Build history of the part. All positions in model axes, mm. Face numbers are marked on the shaded views. Round coordinates to 2 decimals unless told otherwise and drop trailing zeros. Loops run counter-clockwise (first coordinate to the right, second up) from the corner with the lowest first, then second, coordinate; pieces in that order, holes last. Notation, with made-up numbers: (80.5, 28) -> (126.5, 28) arc R26 ccw to (126.5, 46) -> close; hole circle Ø6 at (61, 68). An arc over 180 degrees is marked (long way). Put each result on its own line as item: value. Start each with the question number.
```python
from build123d import *


with BuildPart() as part:
    # 草图1 → 旋转1 (revolve)
    with BuildSketch(Plane.XY):
        with BuildLine():
            Line((-10, 0.5), (-5.524030949, 0.5))
            Line((-5.524030949, 0.5), (-5.170477558, 1.112372436))
            Line((-5.170477558, 1.112372436), (-4.463370777, 1.112372436))
            Line((-4.463370777, 1.112372436), (-4.30697363, 2.9))
            ThreePointArc((-4.30697363, 2.9), (-4.74222381, 3.244464966), (-4.50697363, 3.747213595))
            Line((-4.50697363, 3.747213595), (-4.50697363, 5.071428571))
            Line((-4.50697363, 5.071428571), (-3.918095147, 5.071428571))
            Line((-3.918095147, 5.071428571), (-3, 4.428571429))
            Line((-3, 4.428571429), (-3.340059177, 2.5))
            Line((-3.340059177, 2.5), (-3.840059177, 2.5))
            Line((-3.840059177, 2.5), (-4.058780836, 0))
            Line((-4.058780836, 0), (-10.5, 0))
            Line((-10.5, 0), (-11, 0.5))
            Line((-11, 0.5), (-11, 6.5))
            Line((-11, 6.5), (-10.5, 7))
            Line((-10.5, 7), (-5.170477558, 7))
            Line((-5.170477558, 7), (-5.170477558, 6.5))
            Line((-5.170477558, 6.5), (-10, 6.5))
            Line((-10, 6.5), (-10, 0.5))
        make_face()
    revolve(axis=Axis((0, 5.836193369, 0), (0, -1, 0)))


solid = part.part
```
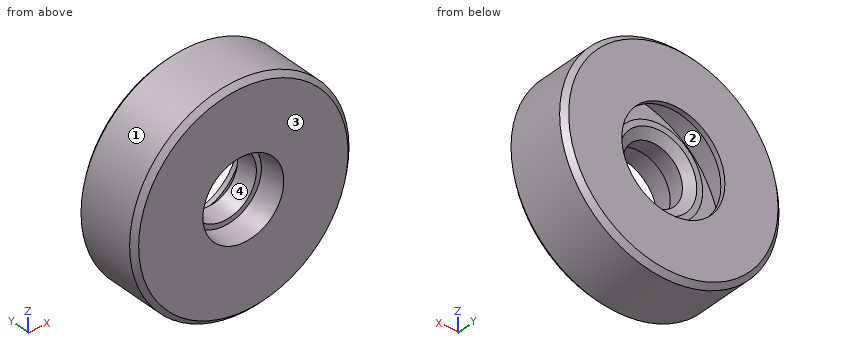
Item 1: Wall check: line 1 (X direction, y = 5.3, z = 0); line 2 (Z direction, x = -4, y = 2.25); line 3 (Y direction, x = 0.25, z = -5.75). Give the ranges that are in metal, low to high. Write a range as from..to.
Item 2: Pull direction Z, two halves, no side cores. Call the marked faces 1, 2, 3 and 4: +Z half, -Z half, draft (parallel to the pull), parting line (faces both ways), or undercut.
Item 3: Drop flat-ended pins along their axis: pin 1 (1.5 mm diameter, centred on y = 4.5, z = 2.5, fed in from -X); pin 2 (1.5 mm diameter, centred on x = 7.5, y = 1.5, fed in from -Z); pin 3 (4 mm diameter, centred on y = 6, z = -2.5, fed in from +X). Give the stop position or say it passes through.
Item 4: Cut at A-A on y = 1.75. Write the cut outline in (x, z), then the cut area to 3 significant figures.
Ans:
1. line 1: x = -11..-10, 10..11
1. line 2: z = -10.25..-9.17, -1.74..1.74, 9.17..10.25
1. line 3: y = 0..0.5, 6.5..7
2. face 1: parting line
2. face 2: undercut
2. face 3: draft
2. face 4: undercut
3. pin 1: stops at x = -10.86
3. pin 2: stops at z = -8.69
3. pin 3: stops at x = 10.99
4. outline: circle Ø22 at (0, 0); circle Ø8.82 at (0, 0); hole circle Ø20 at (0, 0); hole circle Ø7.81 at (0, 0)
4. area: 79.1 mm2
